```python
from build123d import *

# Parameters (mm, degrees)
F1_R     = 1.5
F2_DEPTH = 1.5
F3_DEPTH = 10
F4_DEPTH = 80
F5_R     = 5
F6_R     = 1.49999
F7_R     = 4


# Not quite as in the source:
# - a fillet or chamfer is up to 0.001 mm smaller than in the source, because OpenCascade refuses the exact size
# - a feature names something its author has since deleted; it is built from what else it names


with BuildPart() as f2:
    # F1 (on Top) → F2 (new body)
    with BuildSketch(Plane.XY):
        Polygon((-85, -12.5), (-85, -1.5), (-1.5, -1.5), (-1.5, -12.5), (0, -12.5), (0, 0), (-86.5, 0), (-86.5, -12.5), align=None)
        Polygon((-48.25, -12.5), (-80, -12.5), (-80, -14), (-6.5, -14), (-6.5, -12.5), (-38.25, -12.5), align=None)
        with BuildLine():
            Line((-1.5, -1.5), (-85, -1.5))
            Line((-85, -1.5), (-85, -12.5))
            Line((-85, -12.5), (-80, -12.5))
            Line((-80, -12.5), (-48.25, -12.5))
            ThreePointArc((-48.25, -12.5), (-49.6642135624, -11.9142135624), (-50.25, -10.5))
            Line((-50.25, -10.5), (-50.25, -7.5))
            ThreePointArc((-50.25, -7.5), (-49.6642135624, -6.0857864376), (-48.25, -5.5))
            Line((-48.25, -5.5), (-38.25, -5.5))
            ThreePointArc((-38.25, -5.5), (-36.8357864376, -6.0857864376), (-36.25, -7.5))
            Line((-36.25, -7.5), (-36.25, -10.5))
            ThreePointArc((-36.25, -10.5), (-36.8357864376, -11.9142135624), (-38.25, -12.5))
            Line((-38.25, -12.5), (-6.5, -12.5))
            Line((-6.5, -12.5), (-1.5, -12.5))
            Line((-1.5, -12.5), (-1.5, -1.5))
        make_face()
        with BuildLine():
            Line((-86.5, -14), (-86.5, -12.5))
            Line((-86.5, -12.5), (-86.5, 0))
            Line((-86.5, 0), (-89.5, 0))
            ThreePointArc((-89.5, 0), (-96.5, -7), (-89.5, -14))
            Line((-89.5, -14), (-86.5, -14))
        make_face()
        with Locations((-92, -7)):
            Circle(F1_R, mode=Mode.SUBTRACT)
        with BuildLine():
            Line((0, 0), (0, -12.5))
            Line((0, -12.5), (0, -14))
            Line((0, -14), (3, -14))
            ThreePointArc((3, -14), (10, -7), (3, 0))
            Line((3, 0), (0, 0))
        make_face()
        with Locations((5.5, -7)):
            Circle(F1_R, mode=Mode.SUBTRACT)
        Polygon((-80, -12.5), (-85, -12.5), (-86.5, -12.5), (-86.5, -14), (-80, -14), align=None)
        Polygon((0, -12.5), (-1.5, -12.5), (-6.5, -12.5), (-6.5, -14), (0, -14), align=None)
    extrude(amount=-F2_DEPTH)

    # F1 (on Top) → F3 (join)
    with BuildSketch(Plane.XY):
        Polygon((0, -12.5), (-1.5, -12.5), (-6.5, -12.5), (-6.5, -14), (0, -14), align=None)
        Polygon((-80, -12.5), (-85, -12.5), (-86.5, -12.5), (-86.5, -14), (-80, -14), align=None)
        Polygon((-48.25, -12.5), (-80, -12.5), (-80, -14), (-6.5, -14), (-6.5, -12.5), (-38.25, -12.5), align=None)
    extrude(amount=F3_DEPTH)

    # F1 (on Top) → F4 (join)
    with BuildSketch(Plane.XY):
        Polygon((-85, -12.5), (-85, -1.5), (-1.5, -1.5), (-1.5, -12.5), (0, -12.5), (0, 0), (-86.5, 0), (-86.5, -12.5), align=None)
        Polygon((-80, -12.5), (-85, -12.5), (-86.5, -12.5), (-86.5, -14), (-80, -14), align=None)
        Polygon((0, -12.5), (-1.5, -12.5), (-6.5, -12.5), (-6.5, -14), (0, -14), align=None)
    extrude(amount=F4_DEPTH)

    # F5
    f5_edges = [f2.edges().sort_by_distance(p)[0] for p in [
        (-80, -13.25, 80),
        (-6.5, -13.25, 80),
    ]]
    fillet(f5_edges, radius=F5_R)

    # F6 (radius 1.5 in the source; OpenCascade refuses exactly that, so slightly less here)
    f6_edges = [f2.edges().sort_by_distance(p)[0] for p in [
        (-43.25, -12.5, 10),
        (-86.5, -7, 0),
        (0, -7, 0),
    ]]
    fillet(f6_edges, radius=F6_R)

    # F7
    f7_edges = [f2.edges().sort_by_distance(p)[0] for p in [
        (-85, -1.5, 40),
        (-1.5, -1.5, 40),
    ]]
    fillet(f7_edges, radius=F7_R)


solid = f2.part
```
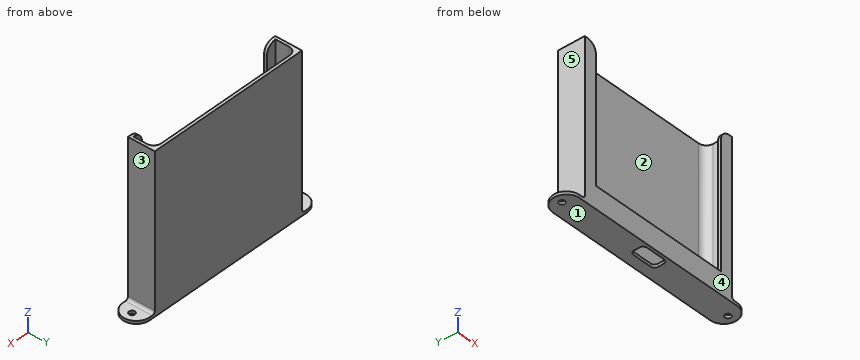
Design review of the part built by this model. Coordinates are the model's own, in mm. Face numbers are marked on the shaded views. A direction names the side the tool comes from. Round coordinates to 2 decimals unless told otherwise and drop trailing zeros. Write each loop counter-clockwise with the first axis right and the second up, starting at its lowest first coordinate (ties: lowest second). Pieces come first, ordered by that corner, then holes.
Item 1: The part is to be moulded in two halves that separate along X. For the marked faces 1, 2 and 3, say which applies: +X half, -X half, draft (parallel to the pull), parting line (faces both ways), or undercut.
Item 2: For probe 1 along X at (y, z) = (-11.25, 59); probe 2 along Z at (x, y) = (-66, -7); probe 3 along X at (y, z) = (-3.5, 25.5), list the stretches that pass through material, from the lowest coordinate up.
Item 3: We need section B-B on z = 6.5. Write out the cut boundary in (x, y), and give its area (3 significant figures).
Item 4: Clearance check with flat-ended pins moving along their axes: pin 1 Ø5 at (y, z) = (-10, 47) entering from -X; pin 2 Ø4 at (y, z) = (-3.5, 65) entering from +X; pin 3 Ø1.8 at (x, y) = (5.5, -7) entering from +Z; pin 4 Ø12 at (x, z) = (-66.5, 67) entering from -Y. State where each tip first meets the part, or that it passes through.
Item 5: We need section C-C on z = 58.5. Write out the cut boundary in (x, y).
Item 6: For the marked faces 4 and 5, list the 3-axis set-ups (+Z, -Z, +X, -X, +Y, -Y) from which the entire face can be reached by the end or side of a thin tool; tool diameter is ignored.
Returned:
1. face 1: draft
1. face 2: undercut
1. face 3: +X half
2. probe 1: x = -86.5 to -85, -1.5 to 0
2. probe 2: z = -1.5 to 0
2. probe 3: x = -86.5 to -84.46, -2.04 to 0
3. outline: (-86.5, -14) - (0, -14) - (0, 0) - (-86.5, 0) - close; hole (-85, -12.5) - (-1.5, -12.5) - (-1.5, -5.5) arc R4 ccw to (-5.5, -1.5) - (-81, -1.5) arc R4 ccw to (-85, -5.5) - close
3. area: 299 mm2
4. pin 1: stops at x = -86.5
4. pin 2: stops at x = 0
4. pin 3: passes through
4. pin 4: stops at y = -1.5
5. outline: (-86.5, -14) - (-80, -14) - (-80, -12.5) - (-85, -12.5) - (-85, -5.5) arc R4 cw to (-81, -1.5) - (-5.5, -1.5) arc R4 cw to (-1.5, -5.5) - (-1.5, -12.5) - (-6.5, -12.5) - (-6.5, -14) - (0, -14) - (0, 0) - (-86.5, 0) - close
6. face 4: +Z, -Z, +X, -X, -Y
6. face 5: +Z, -X, +Y, -Y
